Geometry: final body of the model. Coordinates: model frame, mm. A direction names the side the tool comes from. Round coordinates to 2 decimals unless told otherwise and drop trailing zeros. Loops run counter-clockwise (first coordinate to the right, second up) from the corner with the lowest first, then second, coordinate; pieces in that order, holes last. Notation, with made-up numbers: (-4.5, 64.25) - (10.5, 64.25) arc R20 cw to (10.5, 93.25) - close; hole circle Ø7 at (-13, 30). An arc over 180 degrees is marked (long way). Answer as a JSON object with one key per item and string values. Group by question number.
Item 1: Draft query along Z for faces 1 (the face through (-1.612, 1.482, -2.103)), 2 (the face through (-2, 0, 0)), 3 (the face through (0, 2.5, 1.25)). Return one class per face: released by +Z, released by -Z, zero draft, split by the parting line, or undercut.
Item 2: Line query: line 1 (Z direction, x = -0.4, y = -1.5); line 2 (Y direction, x = 2.15, z = 0.75); line 3 (X direction, y = -21, z = -0.05). Output: solid intervals per line, ascending.
Item 3: First-contact query: pin 1 (0.8 mm diameter, centred on x = -0.5, z = 0.5, fed in from +Y); pin 2 (3 mm diameter, centred on x = -0.5, y = -33.5, fed in from +Z); pin 3 (0.8 mm diameter, centred on x = -0.5, y = 2.5, fed in from +Z). Flat tips, straight axial feed; report the tip coordinate or a pass-through.
Item 4: Reachability of faces 4 (the face through (0, -60, 0)), 5 (the face through (0.45, -29.58, -1.43)), 6 (the face through (1.08, 2.51, 0.63)) from +Z, -Z, +X, -X, +Y, -Y: full face, straight path, thin tool, end or side. Return the list, or none.
Item 5: Section A-A (x = 0). Return the cut outline in (y, z).
Item 6: Section B-B (y = -11.5). Return the cut outline in (x, z).
```python
from build123d import *

# Parameters (mm, degrees)
SKETCH1_R           = 2.65
BOSS_EXTRUDE1_DEPTH = 3
CUT_EXTRUDE1_DEPTH  = 1
SKETCH3_R           = 1.5
BOSS_EXTRUDE2_DEPTH = 60
FILLET1_R           = 0.2


with BuildPart() as part:
    # Sketch1 → Boss-Extrude1 (new body)
    with BuildSketch(Plane(origin=(0, 0, 0), x_dir=(1, 0, 0), z_dir=(0, 1, 0))):
        with Locations(Location((0, 0, 0), (0, 0, 270))):
            Circle(SKETCH1_R)
    extrude(amount=BOSS_EXTRUDE1_DEPTH)

    # Sketch2 → Cut-Extrude1 (cut)
    with BuildSketch(Plane(origin=(0, 3, 0), x_dir=(1, 0, 0), z_dir=(0, 1, 0))):
        Polygon((1.443375673, 0), (0.721687836, 1.25), (-0.721687836, 1.25), (-1.443375673, 0), (-0.721687836, -1.25), (0.721687836, -1.25), align=None)
    extrude(amount=-CUT_EXTRUDE1_DEPTH, mode=Mode.SUBTRACT)

    # Sketch3 → Boss-Extrude2 (add)
    with BuildSketch(Plane.XZ):
        with Locations(Location((0, 0, 0), (0, 0, 270))):
            Circle(SKETCH3_R)
    extrude(amount=BOSS_EXTRUDE2_DEPTH)

    # Fillet1
    fillet1_edges = [part.edges().sort_by_distance(p)[0] for p in [
        (0, 0, -2.65),
        (0, 3, -2.65),
    ]]
    fillet(fillet1_edges, radius=FILLET1_R)


solid = part.part
```
Values:
{
 "1": {"face 1": "split by the parting line", "face 2": "zero draft", "face 3": "undercut"},
 "2": {"line 1": "z = -1.45 to 1.45", "line 2": "y = 0 to 3", "line 3": "x = -1.5 to 1.5"},
 "3": {"pin 1": "stops at y = 2", "pin 2": "stops at z = 1.5", "pin 3": "stops at z = 2.65"},
 "4": {"face 4": "+Z, -Z, +X, -X, -Y", "face 5": "-Y", "face 6": "+Y"},
 "5": {"outline": "(-60, -1.5) - (0, -1.5) - (0, -2.45) arc R0.2 ccw to (0.2, -2.65) - (2.8, -2.65) arc R0.2 ccw to (3, -2.45) - (3, -1.25) - (2, -1.25) - (2, 1.25) - (3, 1.25) - (3, 2.45) arc R0.2 ccw to (2.8, 2.65) - (0.2, 2.65) arc R0.2 ccw to (0, 2.45) - (0, 1.5) - (-60, 1.5) - close"},
 "6": {"outline": "circle Ø3 at (0, 0)"}
}
